```python
from build123d import *

# Parameters (mm, degrees)
P01_STANDOFF_START      = 3
SK_P01_STANDOFF_R       = 1.5
P01_STANDOFF_DEPTH      = 3
P02_STANDOFF_START      = 3
SK_P02_STANDOFF_R       = 1.5
P02_STANDOFF_DEPTH      = 3
P03_VL53L4CDBOARD_START = 1.4
SK_P03_VL53L4CDBOARD_W  = 25.4
SK_P03_VL53L4CDBOARD_H  = 17.78
P03_VL53L4CDBOARD_DEPTH = 1.6
SK_P04_TOFSENSOR_W      = 5
SK_P04_TOFSENSOR_H      = 3
P04_TOFSENSOR_DEPTH     = 1.4


with BuildPart() as part:
    # SK_P01_Standoff → P01_Standoff (new body)
    with BuildSketch(Plane(origin=(0, 0, 0), x_dir=(1, 0, 0), z_dir=(0, 1, 0)).offset(P01_STANDOFF_START)):
        with Locations(Location((-10.16, 6.35, 0), (0, 0, 270))):
            Circle(SK_P01_STANDOFF_R)
    extrude(amount=P01_STANDOFF_DEPTH)



with BuildPart() as body_2:
    # SK_P02_Standoff → P02_Standoff (new body)
    with BuildSketch(Plane(origin=(0, 0, 0), x_dir=(1, 0, 0), z_dir=(0, 1, 0)).offset(P02_STANDOFF_START)):
        with Locations(Location((10.16, -6.35, 0), (0, 0, 270))):
            Circle(SK_P02_STANDOFF_R)
    extrude(amount=P02_STANDOFF_DEPTH)


with BuildPart() as part_1:
    add(part.part)

    add(body_2.part)  # P03_VL53L4CDboard merges body 2
    # SK_P03_VL53L4CDboard → P03_VL53L4CDboard (add)
    with BuildSketch(Plane(origin=(0, 0, 0), x_dir=(1, 0, 0), z_dir=(0, 1, 0)).offset(P03_VL53L4CDBOARD_START)):
        Rectangle(SK_P03_VL53L4CDBOARD_W, SK_P03_VL53L4CDBOARD_H)
    extrude(amount=P03_VL53L4CDBOARD_DEPTH)

    # SK_P04_ToFsensor → P04_ToFsensor (add)
    with BuildSketch(Plane(origin=(0, 0, 0), x_dir=(1, 0, 0), z_dir=(0, 1, 0))):
        Rectangle(SK_P04_TOFSENSOR_W, SK_P04_TOFSENSOR_H)
    extrude(amount=P04_TOFSENSOR_DEPTH)


solid = part_1.part
```
Verification items for the finished model (mm, model axes). A direction names the side the tool comes from. Coordinates: 2 decimals unless noted, no trailing zeros. Loops run counter-clockwise (first coordinate to the right, second up) from the corner with the lowest first, then second, coordinate; pieces in that order, holes last. Notation, with made-up numbers: (59.25, 13.5) - (84.25, 13.5) arc R18 ccw to (84.25, 48.5) - close; hole circle Ø3 at (-17.5, -12.5). An arc over 180 degrees is marked (long way). Return JSON: item names as keys, results as strings.
1. Go/stop test with flat-tipped pins: pin 1 (1.1 mm diameter, centred on x = 0.5, y = 0.5, fed in from +Z); pin 2 (1.5 mm diameter, centred on y = 1, z = 0.5, fed in from -X); pin 3 (0.7 mm diameter, centred on y = 1, z = -0.5, fed in from +X); pin 4 (9 mm diameter, centred on x = -5.5, z = 2, fed in from +Y). Record where each tip stops, or that it passes through.
Established:
{"pin 1": "stops at z = 1.5", "pin 2": "stops at x = -12.7", "pin 3": "stops at x = 2.5", "pin 4": "stops at y = 3"}
2. Thickness scan on L1, parallel to Y at x = -7.5, z = -3.5; L2, parallel to Y at x = 2, z = 1; L3, parallel to Z at x = -10.5, y = 4.2. Record the ranges inside material, lowest first.
Established:
{"L1": "y = 1.4 to 3", "L2": "y = 0 to 3", "L3": "z = -7.81 to -4.89"}
3. Section check D-D, the plane y = 0.85. Record the boundary of the cut face in (x, z), then the cut area to 3 significant figures.
Established:
{"outline": "(-2.5, -1.5) - (2.5, -1.5) - (2.5, 1.5) - (-2.5, 1.5) - close", "area": "15.0 mm2"}
4. Section check A-A, the plane x = -1. Record the boundary of the cut face in (y, z), then the cut area to 3 significant figures.
Established:
{"outline": "(0, -1.5) - (1.4, -1.5) - (1.4, -8.89) - (3, -8.89) - (3, 8.89) - (1.4, 8.89) - (1.4, 1.5) - (0, 1.5) - close", "area": "32.6 mm2"}
5. Section check C-C, the plane y = 3.9. Record the boundary of the cut face in (x, z), then the cut area to 3 significant figures.
Established:
{"outline": "circle Ø3 at (-10.16, -6.35); circle Ø3 at (10.16, 6.35)", "area": "14.1 mm2"}
6. Section check B-B, the plane z = -6.35. Record the boundary of the cut face in (x, y), then the cut area to 3 significant figures.
Established:
{"outline": "(-12.7, 1.4) - (12.7, 1.4) - (12.7, 3) - (-8.66, 3) - (-8.66, 6) - (-11.66, 6) - (-11.66, 3) - (-12.7, 3) - close", "area": "49.6 mm2"}
7. Tool access check on faces 1 (the flat face through (0, 1, 1.5)), 2 (the cylindrical face through (-8.895, 4.479, -5.544)), 3 (the flat face through (0, 1, -1.5)), 4 (the flat face through (-2.5, 1, 0)), 5 (the flat face through (2.5, 1, 0)). Record the directions out of +Z, -Z, +X, -X, +Y, -Y that give a thin tool (end or side, any length) a straight path to the whole face; none if there is none.
Established:
{"face 1": "+Z, +X, -X, -Y", "face 2": "+Y", "face 3": "-Z, +X, -X, -Y", "face 4": "+Z, -Z, -X, -Y", "face 5": "+Z, -Z, +X, -Y"}
